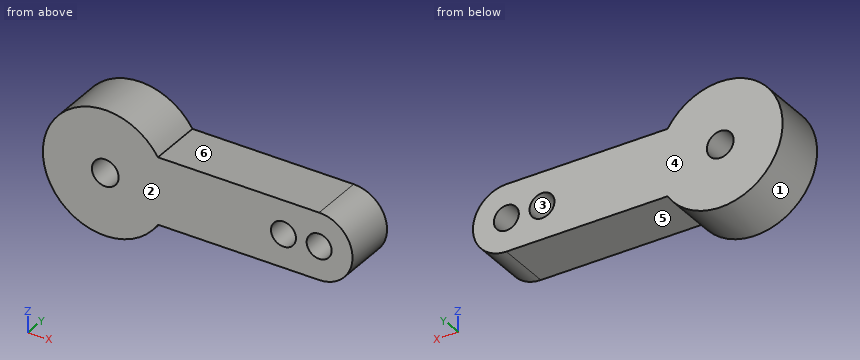
Autodesk Fusion 360 part; units mm, degrees
sketch "Skizze1" plane through (0, 0, 0) normal (0, 1, 0) x (1, 0, 0)
  circle A0 centre (0, 0) radius 1.5
  circle A1 centre (20, 0) radius 1.4
  circle A2 centre (24, 0) radius 1.4
  line L0 (0, 0) -> (24, 0) construction
  line L1 (24, 3.75) -> (5.9108, 3.75)
  line L2 (24, -3.75) -> (5.9108, -3.75)
  arc A3 (24, -3.75) -> (24, 3.75) centre (24, 0) ccw
  arc A4 (5.9108, 3.75) -> (5.9108, -3.75) centre (0, 0) ccw
  dimension "d1" = 3
  dimension "d2" = 2.8
  dimension "d3" = 2.8
  dimension "d4" = 20
  dimension "d5" = 4
  dimension "d6" = 14
  dimension "d7" = 7.5
extrude "Extrusion1" add sketch "Skizze1" along normal blind 6
Could you check a few things on this model? Use its own coordinates, in mm. Face numbers are marked on the shaded views. A direction names the side the tool comes from. Give positions to 0.01 mm unless a question says otherwise; leave off trailing zeros. Order: outer loops, then holes, each group sorted by start corner. A loop starts at its lowest first (then second) coordinate and runs counter-clockwise, first axis right, second up.
Item 1: If we section it at C-C, the plane z = 0: Write out the boundary of the cut face in (x, y).
Item 2: If we section it at B-B, the plane x = 20: Write out the boundary of the cut face in (y, z), plus the area to 3 significant figures.
Item 3: I'm going to push flat-ended pins straight in: pin 1 (1 mm diameter, centred on x = -1.5, y = 4.5, fed in from +Z); pin 2 (3 mm diameter, centred on x = 12.5, y = 3.5, fed in from -Z); pin 3 (2 mm diameter, centred on x = 24, z = 0, fed in from -Y). Where does each tip first touch, or does it pass through?
Item 4: For the marked faces 4, 5 and 6, which set-ups out of +Z, -Z, +X, -X, +Y, -Y let a thin tool reach every point of the face, with its end or its side?
Item 5: If we mould it in two halves opening along Z, with no side actions, what happens to the marked faces 1, 2 and 3? For each: pulls with the +Z half, pulls with the -Z half, needs draft (parallel to the pull), parting line crosses it, or undercut.
Item 6: If we section it at A-A, the plane y = 5.3: Write out the boundary of the cut face in (x, z), plus the area to 3 significant figures.
Item 7: I need wall thicknesses on line 1 (X direction, y = 3, z = 0); line 2 (Z direction, x = 24, y = 2.6); line 3 (X direction, y = 1.05, z = -0.5). Which ranges of each line are inside material? Lowest first, please.
Item 8: If we section it at D-D, the plane x = 0: Write out the boundary of the cut face in (y, z), plus the area to 3 significant figures.
Values:
1. outline: (-7, 0) - (-1.5, 0) - (-1.5, 6) - (-7, 6) - close; (1.5, 0) - (18.6, 0) - (18.6, 6) - (1.5, 6) - close; (21.4, 0) - (22.6, 0) - (22.6, 6) - (21.4, 6) - close; (25.4, 0) - (27.75, 0) - (27.75, 6) - (25.4, 6) - close
2. outline: (0, -3.75) - (6, -3.75) - (6, -1.4) - (0, -1.4) - close; (0, 1.4) - (6, 1.4) - (6, 3.75) - (0, 3.75) - close
2. area: 28.2 mm2
3. pin 1: stops at z = 6.93
3. pin 2: stops at z = -3.75
3. pin 3: passes through
4. face 4: +Z, -Z, +X, -X, +Y
4. face 5: -Z, +X, +Y, -Y
4. face 6: +Z, +X, +Y, -Y
5. face 1: parting line crosses it
5. face 2: needs draft
5. face 3: undercut
6. outline: (5.91, -3.75) - (24, -3.75) arc R3.75 ccw to (24, 3.75) - (5.91, 3.75) arc R7 ccw (long way) to start; hole circle Ø3 at (0, 0); hole circle Ø2.8 at (20, 0); hole circle Ø2.8 at (24, 0)
6. area: 287 mm2
7. line 1: x = -7 to -1.5, 1.5 to 18.6, 21.4 to 22.6, 25.4 to 27.75
7. line 2: z = -3.75 to -1.4, 1.4 to 3.75
7. line 3: x = -6.98 to -1.41, 1.41 to 18.69, 21.31 to 22.69, 25.31 to 27.72
8. outline: (0, -7) - (6, -7) - (6, -1.5) - (0, -1.5) - close; (0, 1.5) - (6, 1.5) - (6, 7) - (0, 7) - close
8. area: 66.0 mm2
